Part model, mm, in its own coordinate system. Face numbers are marked on the shaded views. A direction names the side the tool comes from. Round coordinates to 2 decimals unless told otherwise and drop trailing zeros. Write each loop counter-clockwise with the first axis right and the second up, starting at its lowest first coordinate (ties: lowest second). Pieces come first, ordered by that corner, then holes. Notation, with made-up numbers: M 14.5,58 L 28.5,58 A5 ccw 28.5,67 Z; hole C -17.5,23 d6. An arc over 180 degrees is marked long. Answer as a JSON object with one key per item and string values. Group by question number.
1. Which spindle directions (+Z, -Z, +X, -X, +Y, -Y) get a long thin tool onto all of the face, cutting with end or side? Do the marked faces 4 and 5. Say none if no direction does.
2. Band-saw the part on C-C, the plane y = 5.5. Write the cut outline in (x, z).
3. Drill centre lines: line 1 (X direction, y = 27.65, z = 19.9); line 2 (Z direction, x = 1.45, y = 15); line 3 (Y direction, x = 8, z = 127). Where is each one in solid material? Low to high. Write a range as from..to.
4. Band-saw the part on A-A, the plane z = 116. Write the cut outline in (x, y).
5. Drop flat-ended pins along their axis: pin 1 (5 mm diameter, centred on y = 22, z = 40.5, fed in from -X); pin 2 (2.5 mm diameter, centred on y = 15, z = 116, fed in from +X). Give the stop position or say it passes through.
6. Two-plate mould, pull along Y, no slides. Class the marked faces 1, 2 and 3: +Y half, -Y half, draft (parallel to the pull), parting line (faces both ways), or undercut.
7. Band-saw the part on D-D, the plane x = 32. Write the cut outline in (y, z), plus the area to 3 significant figures.
8. Band-saw the part on B-B, the plane x = 13.5. Write the cut outline in (y, z).
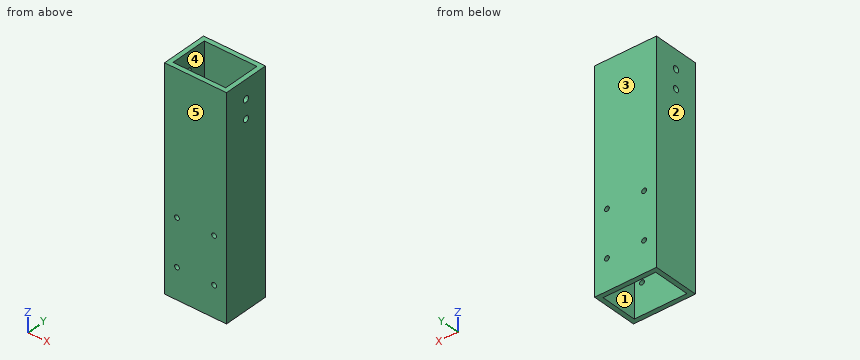
from build123d import *

# Parameters (mm, degrees)
SKETCH_1_W          = 40
SKETCH_1_H          = 30
SKETCH_1_W_2        = 34
SKETCH_1_H_2        = 24
EXTRUDE_1_DEPTH     = 140
SKETCH_2_R          = 2
CUT_EXTRUDE_1_DEPTH = 149.660687473
SKETCH_3_R          = 1.55
CUT_EXTRUDE_2_DEPTH = 149.660687473


with BuildPart() as part:
    # 草图1 → 凸台-拉伸1 (new body)
    with BuildSketch(Plane.XY):
        with Locations((20, 15)):
            Rectangle(SKETCH_1_W, SKETCH_1_H)
        with Locations((20, 15)):
            Rectangle(SKETCH_1_W_2, SKETCH_1_H_2, mode=Mode.SUBTRACT)
    extrude(amount=EXTRUDE_1_DEPTH)

    # 草图2 → 切除-拉伸1 (cut, through all)
    with BuildSketch(Plane(origin=(0, 0, 0), x_dir=(0, 0, -1), z_dir=(1, 0, 0))):
        with Locations(Location((-116, 15, 0), (0, 0, 180))):
            Circle(SKETCH_2_R)
        with Locations(Location((-128, 15, 0), (0, 0, 180))):
            Circle(SKETCH_2_R)
    extrude(amount=CUT_EXTRUDE_1_DEPTH, mode=Mode.SUBTRACT)

    # 草图3 → 切除-拉伸2 (cut, through all)
    with BuildSketch(Plane(origin=(0, 0, 0), x_dir=(1, 0, 0), z_dir=(0, 1, 0))):
        with Locations(Location((8, -19.9, 0), (0, 0, 90))):
            Circle(SKETCH_3_R)
        with Locations(Location((32, -19.9, 0), (0, 0, 90))):
            Circle(SKETCH_3_R)
        with Locations(Location((32, -49.9, 0), (0, 0, 90))):
            Circle(SKETCH_3_R)
        with Locations(Location((8, -49.9, 0), (0, 0, 90))):
            Circle(SKETCH_3_R)
    extrude(amount=CUT_EXTRUDE_2_DEPTH, mode=Mode.SUBTRACT)


solid = part.part
Worked answers:
{
 "1": {"face 4": "+Z, -Z", "face 5": "+Z, -Z, +X, -X, -Y"},
 "2": {"outline": "M 0,0 L 3,0 L 3,140 L 0,140 Z; M 37,0 L 40,0 L 40,140 L 37,140 Z"},
 "3": {"line 1": "x = 0..6.45, 9.55..30.45, 33.55..40", "line 2": "z = 0..114, 118..126, 130..140", "line 3": "y = 0..3, 27..30"},
 "4": {"outline": "M 0,0 L 40,0 L 40,13 L 37,13 L 37,3 L 3,3 L 3,13 L 0,13 Z; M 0,17 L 3,17 L 3,27 L 37,27 L 37,17 L 40,17 L 40,30 L 0,30 Z"},
 "5": {"pin 1": "stops at x = 0", "pin 2": "passes through"},
 "6": {"face 1": "undercut", "face 2": "draft", "face 3": "+Y half"},
 "7": {"outline": "M 0,0 L 3,0 L 3,18.35 L 0,18.35 Z; M 0,21.45 L 3,21.45 L 3,48.35 L 0,48.35 Z; M 0,51.45 L 3,51.45 L 3,140 L 0,140 Z; M 27,0 L 30,0 L 30,18.35 L 27,18.35 Z; M 27,21.45 L 30,21.45 L 30,48.35 L 27,48.35 Z; M 27,51.45 L 30,51.45 L 30,140 L 27,140 Z", "area": "803 mm^2"},
 "8": {"outline": "M 0,0 L 3,0 L 3,140 L 0,140 Z; M 27,0 L 30,0 L 30,140 L 27,140 Z"}
}
